from build123d import *

# Parameters (mm, degrees)
EXTRUDE_1_DEPTH = 26
SKETCH_3_R      = 165
EXTRUDE_2_DEPTH = 149
EXTRUDE_3_DEPTH = 270.5
EXTRUDE_4_DEPTH = 90


with BuildPart() as part:
    # 草圖1 → 填料-伸長1 (new body)
    with BuildSketch(Plane.XY):
        Polygon((-197.5, 137.5), (-137.5, 197.5), (137.5, 197.5), (197.5, 137.5), (197.5, -137.5), (137.5, -197.5), (-137.5, -197.5), (-197.5, -137.5), align=None)
    extrude(amount=EXTRUDE_1_DEPTH)

    # 草圖3 → 填料-伸長2 (add)
    with BuildSketch(Plane.XY.offset(26)):
        Circle(SKETCH_3_R)
    extrude(amount=EXTRUDE_2_DEPTH)

    # 草圖4 → 填料-伸長3 (add)
    with BuildSketch(Plane(origin=(0, 0, 0), x_dir=(0, 0, -1), z_dir=(1, 0, 0))):
        with BuildLine():
            Line((-36, 100), (-149, 100))
            ThreePointArc((-149, 100), (-156.071067812, 97.071067812), (-159, 90))
            Line((-159, 90), (-159, -90))
            ThreePointArc((-159, -90), (-156.071067812, -97.071067812), (-149, -100))
            Line((-149, -100), (-36, -100))
            ThreePointArc((-36, -100), (-28.928932188, -97.071067812), (-26, -90))
            Line((-26, -90), (-26, 90))
            ThreePointArc((-26, 90), (-28.928932188, 97.071067812), (-36, 100))
        make_face()
    extrude(amount=-EXTRUDE_3_DEPTH)

    # 草圖5 → 填料-伸長4 (add)
    with BuildSketch(Plane.ZY.offset(270.5)):
        with BuildLine():
            Line((54.5, 71.5), (130.5, 71.5))
            ThreePointArc((130.5, 71.5), (137.571067812, 68.571067812), (140.5, 61.5))
            Line((140.5, 61.5), (140.5, -61.5))
            ThreePointArc((140.5, -61.5), (137.571067812, -68.571067812), (130.5, -71.5))
            Line((130.5, -71.5), (54.5, -71.5))
            ThreePointArc((54.5, -71.5), (47.428932188, -68.571067812), (44.5, -61.5))
            Line((44.5, -61.5), (44.5, 61.5))
            ThreePointArc((44.5, 61.5), (47.428932188, 68.571067812), (54.5, 71.5))
        make_face()
    extrude(amount=EXTRUDE_4_DEPTH)


solid = part.part
Read the model definition and answer for the solid it produces. Units are mm, in the model's axes. A direction names the side the tool comes from. Give positions to 0.01 mm unless a question says otherwise; leave off trailing zeros. Loops run counter-clockwise (first coordinate to the right, second up) from the corner with the lowest first, then second, coordinate; pieces in that order, holes last. Notation, with made-up numbers: (0.25, -20) - (21.25, -20) arc R11 cw to (21.25, -6) - close; hole circle Ø4 at (-10.5, 26). An arc over 180 degrees is marked (long way). Answer as CSV lines item,"result". Start each with the question number.
1) Which of the six approach directions +Z, -Z, +X, -X, +Y, -Y give full straight-line access (tool end or side, diameter ignored) to faces 1 (the face through (-197.5, -2, 13)), 2 (the face through (-315, -71.5, 93)), 3 (the face through (-270.5, 1, 34))?
2) Each of these flat-tipped pins is pushed along its axis until it touches: pin 1 Ø23 at (x, z) = (-331.5, 77) entering from +Y; pin 2 Ø10 at (y, z) = (-16, 41.5) entering from +X; pin 3 Ø13 at (y, z) = (-29, 18) entering from -X. Where does it stop, or does it pass through?
3) Find section C-C (z = 74). Write down the section's boundary in (x, y), then the cut area to 3 significant figures.
4) Find section A-A (y = 0). Write down the section's boundary in (x, z).
5) Find section D-D (y = 42). Write down the section's boundary in (x, z).
6) Find section B-B (x = -300). Write down the section's boundary in (y, z), then the cut area to 3 significant figures.
7) Straight lines are drawn through the part: L1, parallel to X at y = -91, z = 27.5; L2, parallel to Y at x = -316.5, z = 106; L3, parallel to Z at x = 142.5, y = -111. For each, find the intervals that lie inside material, in ascending order. Write a range as from..to.
Findings below:
1,face 1,"-Z, -X, +Y, -Y"
1,face 2,"+Z, -Z, -X, -Y"
1,face 3,"-X"
2,pin 1,"y = 71.5"
2,pin 2,"x = 164.63"
2,pin 3,"x = -197.5"
3,outline,"(-360.5, -71.5) - (-270.5, -71.5) - (-270.5, -100) - (-131.24, -100) arc R165 ccw (long way) to (-131.24, 100) - (-270.5, 100) - (-270.5, 71.5) - (-360.5, 71.5) - close"
3,area,"122,000 mm^2"
4,outline,"(-360.5, 44.5) - (-270.5, 44.5) - (-270.5, 26) - (-197.5, 26) - (-197.5, 0) - (197.5, 0) - (197.5, 26) - (165, 26) - (165, 175) - (-165, 175) - (-165, 159) - (-270.5, 159) - (-270.5, 140.5) - (-360.5, 140.5) - close"
5,outline,"(-360.5, 44.5) - (-270.5, 44.5) - (-270.5, 26) - (-197.5, 26) - (-197.5, 0) - (197.5, 0) - (197.5, 26) - (159.57, 26) - (159.57, 175) - (-159.57, 175) - (-159.57, 159) - (-270.5, 159) - (-270.5, 140.5) - (-360.5, 140.5) - close"
6,outline,"(-71.5, 54.5) arc R10 ccw to (-61.5, 44.5) - (61.5, 44.5) arc R10 ccw to (71.5, 54.5) - (71.5, 130.5) arc R10 ccw to (61.5, 140.5) - (-61.5, 140.5) arc R10 ccw to (-71.5, 130.5) - close"
6,area,"13,600 mm^2"
7,L1,"-270.5..137.64"
7,L2,"-71.5..71.5"
7,L3,"0..26"
